from build123d import *

# Parameters (mm, degrees)
F0_R     = 13
F0_R_2   = 11.25
F1_DEPTH = 5
F2_DEPTH = 15
F3_SIZE  = 2
F4_R     = 2


with BuildPart() as f1:
    # F0 (on Top) → F1 (new body)
    with BuildSketch(Plane.XY):
        with Locations((-1.525424, 1.90678)):
            Circle(F0_R)
        with Locations((-1.525424, 1.90678)):
            Circle(F0_R_2, mode=Mode.SUBTRACT)
    extrude(amount=F1_DEPTH)

    # F0 (on Top) → F2 (join)
    with BuildSketch(Plane.XY):
        with Locations((-1.525424, 1.90678)):
            Circle(F0_R_2)
    extrude(amount=F2_DEPTH)

    # F3
    f3_edges = [f1.edges().sort_by_distance(p)[0] for p in [
        (-12.775424, 1.90678, 15),
    ]]
    chamfer(f3_edges, length=F3_SIZE)

    # F4
    f4_edges = [f1.edges().sort_by_distance(p)[0] for p in [
        (-14.525424, 1.90678, 0),
    ]]
    fillet(f4_edges, radius=F4_R)


solid = f1.part
The model under review builds one solid part; all positions refer to its coordinate system, in mm. A direction names the side the tool comes from. Give positions to 0.01 mm unless a question says otherwise; leave off trailing zeros. Order: outer loops, then holes, each group sorted by start corner. A loop starts at its lowest first (then second) coordinate and runs counter-clockwise, first axis right, second up. Notation, with made-up numbers: M 77.5,73.25 L 84.5,73.25 A24 cw 84.5,110.25 Z; hole C 54.5,-30 d9. An arc over 180 degrees is marked long. Answer in a Markdown table with one row per item. Add a question column.
1. Machinability: for faces 1 (the flat face through (-7, 12, 5)), 2 (the flat face through (-2, 2, 0)), which of the approach directions +Z, -Z, +X, -X, +Y, -Y give a long, thin tool a straight path to every point of the face, cutting with its end or side? Answer none if there is none.
2. For pin 1 Ø10 at (x, y) = (-9, 10) entering from +Z; pin 2 Ø1.5 at (y, z) = (9, 13) entering from -X; pin 3 Ø4 at (y, z) = (5.5, 5.5) entering from -X; pin 4 Ø1 at (y, z) = (-4, 9) entering from +X, all flat-tipped, find the tip position at first contact; note any pin that passes through.
3. To check wall thickness, follow line 1 along X through (y, z) = (-7, 13.5); line 2 along X through (y, z) = (10, 6.5); line 3 along Y through (x, z) = (-10, 2.75). State the ranges of each line that lie inside material, in increasing order.
4. Add section A-A on z = 4.5. State the section outline as (x, y) points.
5. Add section B-B on z = 11.5. State the section outline as (x, y) points, plus the area to 3 significant figures.
The answers:
| question | item | result |
|---|---|---|
| 1 | face 1 | +Z |
| 1 | face 2 | -Z, +X, -X, +Y, -Y |
| 2 | pin 1 | z = 15 |
| 2 | pin 2 | x = -10.82 |
| 2 | pin 3 | x = -14.42 |
| 2 | pin 4 | x = 8.34 |
| 3 | line 1 | -7.54 to 4.49 |
| 3 | line 2 | -9.34 to 6.29 |
| 3 | line 3 | -7.95 to 11.76 |
| 4 | outline | C -1.53,1.91 d26 |
| 5 | outline | C -1.53,1.91 d22.5 |
| 5 | area | 398 mm2 |
